Input: part model. Units: mm. Frame: model coordinates. A direction names the side the tool comes from. Coordinates: 2 decimals unless noted, no trailing zeros. Write each loop counter-clockwise with the first axis right and the second up, starting at its lowest first coordinate (ties: lowest second). Pieces come first, ordered by that corner, then holes. Notation, with made-up numbers: M 34,32.5 L 83,32.5 A10 ccw 83,36.5 Z; hole C -25,-30 d3. An arc over 180 degrees is marked long. Answer as a JSON object with one key per item and string values. Group by question number.
from build123d import *

# Parameters (mm, degrees)
SKETCH1_R           = 2.125
SKETCH1_R_2         = 3
BOSS_EXTRUDE1_DEPTH = 12
SKETCH2_W           = 40
SKETCH2_H           = 4
SLOT1_CUT_DEPTH     = 15
SKETCH3_W           = 30
SKETCH3_H           = 4
SLOT2_CUT_DEPTH     = 138.569073559
CUT_EXTRUDE3_DEPTH  = 140.665672232
SKETCH5_W           = 6
SKETCH5_H           = 4
BOSS_EXTRUDE2_DEPTH = 4
CUT_EXTRUDE4_DEPTH  = 4
SKETCH7_W           = 2.5
SKETCH7_H           = 12
BOSS_EXTRUDE3_DEPTH = 1
CUT_EXTRUDE5_DEPTH  = 140.665672232


with BuildPart() as part:
    # Sketch1 → Boss-Extrude1 (new body)
    with BuildSketch(Plane(origin=(0, 0, 0), x_dir=(1, 0, 0), z_dir=(0, 1, 0))):
        with BuildLine():
            Line((0, -7.5), (10, -7.5))
            Line((10, -7.5), (10, -22.5))
            Line((10, -22.5), (60, -22.5))
            Line((60, -22.5), (80.52220172, -42.5))
            Line((80.52220172, -42.5), (125, -42.5))
            ThreePointArc((125, -42.5), (132.5, -35), (125, -27.5))
            Line((125, -27.5), (89, -27.5))
            Line((89, -27.5), (89, 2.5))
            Line((89, 2.5), (41.141232585, 2.5))
            Line((41.141232585, 2.5), (30.480824737, 7.5))
            Line((30.480824737, 7.5), (0, 7.5))
            ThreePointArc((0, 7.5), (-7.5, 0), (0, -7.5))
        make_face()
        with Locations(Location((0, 0, 0), (0, 0, 270))):
            Circle(SKETCH1_R, mode=Mode.SUBTRACT)
        with Locations(Location((125, -35, 0), (0, 0, 270))):
            Circle(SKETCH1_R, mode=Mode.SUBTRACT)
        with Locations(Location((54, -10, 0), (0, 0, 270))):
            Circle(SKETCH1_R_2, mode=Mode.SUBTRACT)
    extrude(amount=BOSS_EXTRUDE1_DEPTH)

    # Sketch2 → Slot1 Cut (cut)
    with BuildSketch(Plane(origin=(0, 0, -7.5), x_dir=(-1, 0, 0), z_dir=(0, 0, -1))):
        with Locations((-12.5, 6)):
            Rectangle(SKETCH2_W, SKETCH2_H)
    extrude(amount=-SLOT1_CUT_DEPTH, mode=Mode.SUBTRACT)

    # Sketch3 → Slot2 Cut (cut, through all)
    with BuildSketch(Plane(origin=(0, 0, 27.5), x_dir=(-1, 0, 0), z_dir=(0, 0, -1))):
        with Locations((-117.5, 6)):
            Rectangle(SKETCH3_W, SKETCH3_H)
    extrude(amount=-SLOT2_CUT_DEPTH, mode=Mode.SUBTRACT)

    # Sketch4 → Cut-Extrude3 (cut, through all)
    with BuildSketch(Plane(origin=(0, 12, 0), x_dir=(1, 0, 0), z_dir=(0, 1, 0))):
        Polygon((10, -19.5), (10, -22.5), (25, -22.5), align=None)
        Polygon((44, 2.5), (89, 2.5), (89, -2.5), align=None)
    extrude(amount=-CUT_EXTRUDE3_DEPTH, mode=Mode.SUBTRACT)

    # Sketch5 → Boss-Extrude2 (add)
    with BuildSketch(Plane(origin=(89, 0, 0), x_dir=(0, 0, -1), z_dir=(1, 0, 0))):
        with Locations((-20, 6)):
            Rectangle(SKETCH5_W, SKETCH5_H)
    extrude(amount=BOSS_EXTRUDE2_DEPTH)

    # Sketch6 → Cut-Extrude4 (cut)
    with BuildSketch(Plane(origin=(0, 8, 0), x_dir=(1, 0, 0), z_dir=(0, 1, 0))):
        with BuildLine():
            Line((91, -23), (89, -23))
            Line((89, -23), (89, -19.5))
            ThreePointArc((89, -19.5), (89.146446609, -19.146446609), (89.5, -19))
            Line((89.5, -19), (90.5, -19))
            ThreePointArc((90.5, -19), (90.853553391, -19.146446609), (91, -19.5))
            Line((91, -19.5), (91, -23))
        make_face()
        with BuildLine():
            Line((91, -17), (93, -17))
            Line((93, -17), (93, -19))
            ThreePointArc((93, -19), (92.414213562, -17.585786438), (91, -17))
        make_face()
    extrude(amount=-CUT_EXTRUDE4_DEPTH, mode=Mode.SUBTRACT)

    # Sketch7 → Boss-Extrude3 (add)
    with BuildSketch(Plane.ZY.offset(-10)):
        with Locations((16.5, 6)):
            Rectangle(SKETCH7_W, SKETCH7_H)
    extrude(amount=BOSS_EXTRUDE3_DEPTH)

    # Sketch8 → Cut-Extrude5 (cut, through all)
    with BuildSketch(Plane(origin=(0, 12, 0), x_dir=(1, 0, 0), z_dir=(0, 1, 0))):
        Polygon((9, -16.5), (10, -15.25), (9, -15.25), align=None)
        Polygon((10, -17.75), (9, -16.5), (9, -17.75), align=None)
    extrude(amount=-CUT_EXTRUDE5_DEPTH, mode=Mode.SUBTRACT)


solid = part.part
Q1. Draft query along Y for faces 4 (the flat face through (91, 6, 21)), 5 (the flat face through (13, 8, 0)), 6 (the flat face through (62, 0, 17)). Return one class per face: released by +Y, released by -Y, zero draft, split by the parting line, or undercut.
Q2. Section D-D, the plane x = 54. Return the cut outline in (y, z), and give its area (3 significant figures).
Q3. Section C-C, the plane z = 10. Return the cut outline in (x, y).
Q4. Access query for faces 1 (the flat face through (10, 6, 11)), 2 (the flat face through (42, 6, 22.5)), 3 (the flat face through (91, 8, 19)). Directions: +Z, -Z, +X, -X, +Y, -Y. A direction counts if a zero-diameter tool reaches every point of the face in a straight line with its end or side. Return the directions, or none.
Q5. Line query: line 1 (Z direction, x = 0, y = 10.3) (3 decimals); line 2 (X direction, y = 8.5, z = 10); line 3 (X direction, y = 1.75, z = 35) (3 decimals). Output: solid intervals per line, ascending. Write a range as from..to.
Q6. Section B-B, the plane y = 6.75. Return the cut outline in (x, z).
Q7. Pin query (flat end, axial travel): pin 1 Ø1 at (x, y) = (99.5, 9.5) entering from -Z; pin 2 Ø1 at (x, y) = (67.5, 7.5) entering from +Z; pin 3 Ø1.2 at (x, y) = (5.5, 11) entering from +Z. Return the tip coordinate at first contact, or that it passes through.
Q8. Section A-A, the plane z = 0. Return the cut outline in (x, y) (3 decimals), and give its area (3 significant figures).
Filled in:
{
 "1": {"face 4": "zero draft", "face 5": "undercut", "face 6": "released by -Y"},
 "2": {"outline": "M 0,-1.39 L 12,-1.39 L 12,7 L 0,7 Z; M 0,13 L 12,13 L 12,22.5 L 0,22.5 Z", "area": "215 mm^2"},
 "3": {"outline": "M 10,0 L 51,0 L 51,12 L 10,12 Z; M 57,0 L 89,0 L 89,12 L 57,12 Z"},
 "4": {"face 1": "-X, +Y, -Y", "face 2": "+Z, -X, +Y, -Y", "face 3": "-Z, +X, +Y"},
 "5": {"line 1": "-7.5..-2.125, 2.125..7.5", "line 2": "10..51, 57..89", "line 3": "72.826..122.875, 127.125..132.5"},
 "6": {"outline": "M 9,16.5 L 10,15.25 L 10,7.5 L 32.5,7.5 L 32.5,-6.55 L 41.14,-2.5 L 44,-2.5 L 89,2.5 L 89,17 L 91,17 A2 ccw 93,19 L 93,23 L 91,23 L 91,19.5 A0.5 cw 90.5,19 L 89.5,19 A0.5 cw 89,19.5 L 89,27.5 L 102.5,27.5 L 102.5,42.5 L 80.52,42.5 L 60,22.5 L 25,22.5 L 10,19.5 L 10,17.75 Z; hole C 54,10 d6"},
 "7": {"pin 1": "z = 27.5", "pin 2": "z = 30.3", "pin 3": "z = 7.5"},
 "8": {"outline": "M -7.5,0 L -2.125,0 L -2.125,4 L -7.5,4 Z; M -7.5,8 L -2.125,8 L -2.125,12 L -7.5,12 Z; M 2.125,0 L 66.5,0 L 66.5,12 L 2.125,12 L 2.125,8 L 32.5,8 L 32.5,4 L 2.125,4 Z", "area": "694 mm^2"}
}
